Source: CAD feature listing. Evaluate the final solid. Frame: model axes, mm. A direction names the side the tool comes from. Round coordinates to 2 decimals unless told otherwise and drop trailing zeros. Order: outer loops, then holes, each group sorted by start corner. A loop starts at its lowest first (then second) coordinate and runs counter-clockwise, first axis right, second up. Notation, with made-up numbers: M 23,81 L 76,81 A18 ccw 76,114 Z; hole C 83,35 d3. An arc over 180 degrees is marked long. Use CSV: the item, a comma, the result in double quotes. Start each with the question number.
Autodesk Inventor part; units mm, degrees
ref_plane "Work Plane1" through (29, 0, 0) normal (0, -1, 0) x (1, 0, 0)
ref_plane "YZ Plane" through (0, 0, 0) normal (1, 0, 0) x (0, 1, 0)
ref_plane "XZ Plane" through (0, 0, 0) normal (0, 1, 0) x (-1, 0, 0)
sketch "Sketch1" plane through (0, 0, 0) normal (0, 0, 1) x (1, 0, 0)
  line L0 (-0.7535, 0) -> (22.225, 0)
  line L1 (22.225, 0) -> (22.225, 1.4224)
  line L2 (22.225, 1.4224) -> (1.5877, 1.4224)
  line L3 (1.5877, 1.4224) -> (0.0001, 1.4224)
  line L4 (0.0001, 1.4224) -> (0, 1.4224)
  line L5 (0, 1.4224) -> (0, 2.3241)
  line L6 (0, 2.3241) -> (-2.8448, 2.3241)
  line L7 (-2.8448, 2.3241) -> (-2.8448, 1.3785)
  line L8 (-2.8448, 1.3785) -> (-1.5494, 1.3785)
  line L9 (-1.5494, 1.3785) -> (-0.7535, 0)
  line L10 (-7.8588, 0) -> (27.239, 0)
  line L11 (0, -0.4648) -> (0, 2.7889)
  line L12 (1.5877, 1.4224) -> (0, 1.4224) construction
  dimension "d1" = 20.6373
  dimension "d2" = 1.5876
  dimension "d3" = 2.8448
  dimension "d4" = 1.2954
  dimension "d5" = 60
  dimension "d6" = 2.8448
  dimension "d7" = 2.8448
  dimension "d8" = 2.757
  dimension "d9" = 4.6482
  dimension "d26" = 22.225
revolve "Body" add sketch "Sketch1" angle 360 about axis through (-0.7535, 0, 0) along (1, 0, 0)
sketch "Sketch2" plane through (-2.8448, 0, 0) normal (-1, 0, 0) x (0, 0, 1)
  circle A0 centre (0, 0) radius 1.3785
  line L0 (0, -3.2537) -> (0, 3.2537)
  line L1 (-3.2537, 0) -> (3.2537, 0)
  line L2 (1.3785, 0) -> (0.6892, -1.1938)
  line L3 (0.6892, -1.1938) -> (-0.6892, -1.1938)
  line L4 (-0.6892, -1.1938) -> (-1.3785, 0)
  line L5 (-1.3785, 0) -> (-0.6892, 1.1938)
  line L6 (-0.6892, 1.1938) -> (0.6892, 1.1938)
  line L7 (0.6892, 1.1938) -> (1.3785, 0)
extrude "Slot" add sketch "Sketch2" against normal up to next contours L7 A0 | A0 L2 | L6 L0 A0 | A0 L0 L3 | L0 L6 A0 | A0 L3 L0 | L4 A0 | A0 L5
fillet "Fillet1" radius 0.2286 1 edges at (-2.8448, -2.3241, 0)
thread "Thread"
chamfer "Chamfer1" distance 0.3785 distance2 0.3785 1 edges at (22.225, -1.4224, 0) measured on face at (22.225, -0.0669, -0.3902)
ref_plane "Work Plane1" through (29, 0, 0) normal (0, -1, 0) x (1, 0, 0)
fillet "Fillet2" radius 0.1016 1 edges at (0.0001, -1.4224, 0)
equation "\"d1\" = GEL"
equation "\"d3\" = KOH"
equation "\"d4\" = INTI"
equation "\"d6\" = GD"
equation "\"d7\" = BDM"
equation "\"d8\" = 1.1547 * SW"
equation "\"d9\" = KOD"
equation "\"d26\" = NLG"
equation "\"d30\" = R"
equation "\"d17\" = RR"
equation "\"d13\" = GEL"
equation "\"d15\" = -0.5 * SPD + 0.5 * GD"
equation "\"d16\" = GUL"
equation "\"GD\" = 2.8448"
equation "\"NLG\" = 22.225"
equation "\"GEL\" = 20.6373"
equation "\"KOD\" = 4.6482"
equation "\"KOH\" = 2.8448"
equation "\"INTI\" = 1.2954"
equation "\"GAL\" = 1.5875"
equation "\"GUL\" = 0.37846"
equation "\"BDM\" = 2.8448"
equation "\"SW\" = 2.3876"
equation "\"RR\" = 0.2286"
equation "\"SPD\" = 2.08788"
equation "\"R\" = 0.1016"
equation "\"PHH\" = 0.127"
equation "\"GD1\" = SPD"
equation "\"THREADDIA\" = 2.8448"
equation "\"FAWI\" = 45deg"
equation "\"KOH1\" = 2.5654"
equation "\"NND\" = 2.8448"
equation "\"TOA\" = 30deg"
equation "\"E0\" = 1.155 * SW"
properties part number "ANSI B18.3 - No. 4 - 40 UNC - 7/8 HS HCS"
(1) Line query: line 1 along X through (y, z) = (-1.4, -0.65); line 2 along Z through (x, y) = (-0.5, -0.4); line 3 along X through (y, z) = (-0.3, 0.85) (3 decimals). Output: solid intervals per line, ascending.
(2) Draft query along Y for faces 4 (the face through (10.82, -0.31, 1.39)), 5 (the face through (-2.154, 0.605, 1.029)), 6 (the face through (-2.845, -1, 1)). Return one class per face: pulls with the +Y half, pulls with the -Y half, needs draft (parallel to the pull), parting line crosses it, or undercut.
(3) Contact query for flat-ended pins moving along their axis: P1, Ø1, axis at x = 15, y = -1, coming from the +Z side; P2, Ø2, axis at x = 3.5, y = -1, coming from the -Z side; P3, Ø2, axis at x = 10.5, y = 2, coming from the -Z side. Output: stop coordinate, or through.
(4) Section A-A on x = 11.5. Return loops of the section in (y, z), plus the area to 3 significant figures.
(5) Reachability of faces 1 (the face through (0, 2, 0)), 2 (the face through (-2, 1.194, 0)), 3 (the face through (-1.33, -0.5, 2.27)) from +Z, -Z, +X, -X, +Y, -Y: full face, straight path, thin tool, end or side. Return the list, or none.
Results below:
1,line 1,"x = -2.84 to 0"
1,line 2,"z = -2.29 to 2.29"
1,line 3,"x = -1.274 to 22.225"
2,face 4,"parting line crosses it"
2,face 5,"undercut"
2,face 6,"needs draft"
3,P1,"stops at z = 1.33"
3,P2,"stops at z = -1.42"
3,P3,"stops at z = -1.01"
4,outline,"C 0,0 d2.84"
4,area,"6.36 mm2"
5,face 1,"+X"
5,face 2,"-X"
5,face 3,"+X, -X"
